Work out the finished part from the listing and answer in its coordinate system (mm). A direction names the side the tool comes from. Round coordinates to 2 decimals unless told otherwise and drop trailing zeros. Order: outer loops, then holes, each group sorted by start corner. A loop starts at its lowest first (then second) coordinate and runs counter-clockwise, first axis right, second up. Notation, with made-up numbers: (-17, -15.75) - (-12, -15.75) arc R19 ccw to (-12, 11.25) - close; hole circle Ø11 at (-34, -23). An arc over 180 degrees is marked (long way). Use CSV: the item, a comma, the result in double quotes.
from build123d import *

# Parameters (mm, degrees)
F0_R     = 3.45
F1_DEPTH = 1.8
F2_DEPTH = 3.9
F3_R     = 0.3


with BuildPart() as f1:
    # F0 (on Top) → F1 (new body)
    with BuildSketch(Plane.XY):
        with BuildLine():
            Line((56.55, 6.25), (4.145781, 6.25))
            ThreePointArc((4.145781, 6.25), (-7.5, 0), (4.145781, -6.25))
            Line((4.145781, -6.25), (56.55, -6.25))
            Line((56.55, -6.25), (62.8, 0))
            Line((62.8, 0), (56.55, 6.25))
        make_face()
        Circle(F0_R, mode=Mode.SUBTRACT)
    extrude(amount=F1_DEPTH)

    # F0 (on Top) → F2 (join)
    with BuildSketch(Plane.XY):
        Circle(F0_R)
        Polygon((2.580316, -0.319324), (1.598763, -2.050355), (-0.319324, -2.580316), (-2.050355, -1.598763), (-2.580316, 0.319324), (-1.598763, 2.050355), (0.319324, 2.580316), (2.050355, 1.598763), align=None, mode=Mode.SUBTRACT)
    extrude(amount=F2_DEPTH)

    # F3
    f3_edges = [f1.edges().sort_by_distance(p)[0] for p in [
        (-7.5, 0, 1.8),
        (30.34789, 6.25, 1.8),
        (30.34789, -6.25, 1.8),
        (59.675, -3.125, 1.8),
        (59.675, 3.125, 1.8),
        (-7.5, 0, 0),
        (30.34789, -6.25, 0),
        (59.675, 3.125, 0),
        (59.675, -3.125, 0),
        (30.34789, 6.25, 0),
    ]]
    fillet(f3_edges, radius=F3_R)


solid = f1.part
(1) Find section B-B (x = 42). Determine the outline of the cut face in (y, z).
Findings below:
outline,"(-6.25, 0.3) arc R0.3 ccw to (-5.95, 0) - (5.95, 0) arc R0.3 ccw to (6.25, 0.3) - (6.25, 1.5) arc R0.3 ccw to (5.95, 1.8) - (-5.95, 1.8) arc R0.3 ccw to (-6.25, 1.5) - close"
(2) For faces 1 (the flat face through (1.5, -2.3, 3.9)), 2 (the flat face through (-2.1, 1.17, 1.92)), 3 (the cylindrical face through (-0.45, 3.42, 2.84)), 4 (the flat face through (31, 6.25, 1)), 5 (the cylindrical face through (59.567, 3.105, 1.714)), determine the directions among +Z, -Z, +X, -X, +Y, -Y from which every point of the face is accessible in a straight line to the end or side of a thin tool.
Findings below:
face 1,"+Z, +X, -X, +Y, -Y"
face 2,"+Z, -Z"
face 3,"+Z"
face 4,"+Z, -Z, +X, +Y"
face 5,"+Z, +X, +Y"
(3) Find section A-A (z = 3.15). Determine the outline of the cut face in (x, y).
Findings below:
outline,"circle Ø6.9 at (0, 0); hole (-2.58, 0.32) - (-2.05, -1.6) - (-0.32, -2.58) - (1.6, -2.05) - (2.58, -0.32) - (2.05, 1.6) - (0.32, 2.58) - (-1.6, 2.05) - close"
(4) Each of these flat-tipped pins is pushed along its axis until it touches: pin 1 (1 mm diameter, centred on x = 38.5, z = 0.5, fed in from -Y); pin 2 (7 mm diameter, centred on x = 38.5, y = 1.5, fed in from +Z); pin 3 (1.5 mm diameter, centred on x = 30, z = 2, fed in from +Y). Where does it stop, or does it pass through?
Findings below:
pin 1,"stops at y = -6.25"
pin 2,"stops at z = 1.8"
pin 3,"stops at y = 6.25"
(5) The mould has two halves that part along X. Classify faces 6 (the flat face through (59.6, -3.2, 0.9)), 7 (the flat face through (2.3, 0.7, 1.9)), 8 (the flat face through (30, -6.25, 1)): released by +X, released by -X, zero draft, split by the parting line, or undercut.
Findings below:
face 6,"released by +X"
face 7,"undercut"
face 8,"zero draft"
(6) Find the intervals of material crossed by L1, parallel to Y at x = 36.5, z = 0.9; L2, parallel to Z at x = 10.5, y = -2.25; L3, parallel to X at y = -1, z = 2.1, in increasing order. Write a range as from..to.
Findings below:
L1,"y = -6.25..6.25"
L2,"z = 0..1.8"
L3,"x = -3.3..-2.22, 2.19..3.3"
